Verification items for the finished model (mm, model axes). Face numbers are marked on the shaded views. A direction names the side the tool comes from. Round coordinates to 2 decimals unless told otherwise and drop trailing zeros. Write each loop counter-clockwise with the first axis right and the second up, starting at its lowest first coordinate (ties: lowest second). Pieces come first, ordered by that corner, then holes. Notation, with made-up numbers: M 29.5,42.5 L 41.5,42.5 A17 ccw 41.5,65.5 Z; hole C 60,-10.5 d2. An arc over 180 degrees is marked long. Answer in a Markdown table with one row per item. Add a question column.
1. Sectioned sample at A-A on x = 23. Record the cut outline in (y, z) (3 decimals).
2. Sectioned sample at D-D on y = 3.5. Record the cut outline in (x, z) (3 decimals), plus the area to 3 significant figures.
3. Draft check along Y on the marked faces 3, 4 and 5. Enter one of: pulls with the +Y half, pulls with the -Y half, needs draft (parallel to the pull), parting line crosses it, or undercut.
4. Set-up check for the marked faces 1 and 2: record each of +Z, -Z, +X, -X, +Y, -Y from which the full face is reachable in a straight line by a thin tool's end or side.
5. Go/stop test with flat-tipped pins: pin 1 Ø1 at (x, z) = (13, 2) entering from +Y; pin 2 Ø1.5 at (x, z) = (28, 2.5) entering from -Y. Record where each tip stops, or that it passes through.
6. Material ranges on probe 1 along Y at (x, z) = (23, 2.55); probe 2 along X at (y, z) = (-0.75, 2); probe 3 along Y at (x, z) = (6.5, 3), recorded low to high.
7. Sectioned sample at C-C on x = 32. Record the cut outline in (y, z) (3 decimals).
8. Sectioned sample at B-B on z = 1.95. Count the separate pieces of the cut face and the enclosed holes in it, plus the area to 3 significant figures.
```python
from build123d import *

# Parameters (mm, degrees)
F0_R     = 1.6
F1_DEPTH = 3.175


# Not quite as in the source:
# - a feature names something its author has since deleted; it is built from what else it names


with BuildPart() as f1:
    # F0 (on Top) → F1 (new body)
    with BuildSketch(Plane.XY):
        with BuildLine():
            Line((32.6, 5), (5.5901699437, 5))
            ThreePointArc((5.5901699437, 5), (-7.5, 0), (5.5901699437, -5))
            Line((5.5901699437, -5), (32.6, -5))
            ThreePointArc((32.6, -5), (36.1355339059, -3.5355339059), (37.6, 0))
            ThreePointArc((37.6, 0), (36.1355339059, 3.5355339059), (32.6, 5))
        make_face()
        Polygon((-0.4246363361, 2.7189872831), (-0.0526366882, 2.4335419138), (0.3193629596, 2.7189872831), (0.6048083289, 2.3469876353), (1.038011094, 2.5264260959), (1.2174495546, 2.0932233308), (1.6823333844, 2.154426448), (1.7435365017, 1.6895426182), (2.2084203316, 1.6283395009), (2.1472172143, 1.163455671), (2.5804199794, 0.9840172105), (2.4009815188, 0.5508144453), (2.7729811667, 0.265369076), (2.4875357974, -0.1066305718), (2.7729811667, -0.4786302196), (2.4009815188, -0.7640755889), (2.5804199794, -1.197278354), (2.1472172143, -1.3767168146), (2.2084203316, -1.8416006445), (1.7435365017, -1.9028037618), (1.6823333844, -2.3676875916), (1.2174495546, -2.3064844743), (1.038011094, -2.7396872394), (0.6048083289, -2.5602487789), (0.3193629596, -2.9322484267), (-0.0526366882, -2.6468030574), (-0.4246363361, -2.9322484267), (-0.7100817054, -2.5602487789), (-1.1432844705, -2.7396872394), (-1.322722931, -2.3064844743), (-1.7876067609, -2.3676875916), (-1.8488098782, -1.9028037618), (-2.3136937081, -1.8416006445), (-2.2524905908, -1.3767168146), (-2.6856933559, -1.197278354), (-2.5062548953, -0.7640755889), (-2.8782545432, -0.4786302196), (-2.5928091739, -0.1066305718), (-2.8782545432, 0.265369076), (-2.5062548953, 0.5508144453), (-2.6856933559, 0.9840172105), (-2.2524905908, 1.163455671), (-2.3136937081, 1.6283395009), (-1.8488098782, 1.6895426182), (-1.7876067609, 2.154426448), (-1.322722931, 2.0932233308), (-1.1432844705, 2.5264260959), (-0.7100817054, 2.3469876353), align=None, mode=Mode.SUBTRACT)
        with Locations((13, 0)):
            Circle(F0_R, mode=Mode.SUBTRACT)
        with Locations((23, 0)):
            Circle(F0_R, mode=Mode.SUBTRACT)
        with Locations((33, 0)):
            Circle(F0_R, mode=Mode.SUBTRACT)
    extrude(amount=F1_DEPTH)


solid = f1.part
```
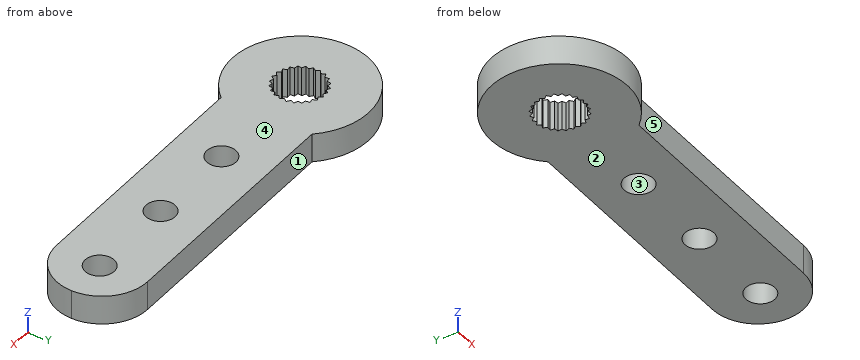
Geometry check:
| question | item | result |
|---|---|---|
| 1 | outline | M -5,0 L -1.6,0 L -1.6,3.175 L -5,3.175 Z; M 1.6,0 L 5,0 L 5,3.175 L 1.6,3.175 Z |
| 2 | outline | M -6.633,0 L 36.171,0 L 36.171,3.175 L -6.633,3.175 Z |
| 2 | area | 136 mm2 |
| 3 | face 3 | undercut |
| 3 | face 4 | needs draft |
| 3 | face 5 | pulls with the -Y half |
| 4 | face 1 | +Z, -Z, +X, +Y |
| 4 | face 2 | -Z, +X, -X, +Y, -Y |
| 5 | pin 1 | stops at y = 5 |
| 5 | pin 2 | stops at y = -5 |
| 6 | probe 1 | y = -5 to -1.6, 1.6 to 5 |
| 6 | probe 2 | x = -7.46 to -2.52, 2.42 to 11.59, 14.41 to 21.59, 24.41 to 31.59, 34.41 to 37.54 |
| 6 | probe 3 | y = -5 to 5 |
| 7 | outline | M -5,0 L -1.249,0 L -1.249,3.175 L -5,3.175 Z; M 1.249,0 L 5,0 L 5,3.175 L 1.249,3.175 Z |
| 8 | separate pieces | 1 |
| 8 | enclosed holes | 4 |
| 8 | area | 426 mm2 |
